Geometry check sheet. Reference: the model listing, model coordinates, mm. Face numbers are marked on the shaded views. A direction names the side the tool comes from. Round coordinates to 2 decimals unless told otherwise and drop trailing zeros. Order: outer loops, then holes, each group sorted by start corner. A loop starts at its lowest first (then second) coordinate and runs counter-clockwise, first axis right, second up. Notation, with made-up numbers: (41, 63.25) - (84, 63.25) arc R16 cw to (84, 77.25) - close; hole circle Ø1 at (62.5, 80). An arc over 180 degrees is marked (long way). Return JSON: item names as keys, results as strings. Group by question number.
Q1. Sectioned sample at C-C, the plane y = -12. Record the cut outline in (x, z).
Q2. Gauge pin test, flat ends, axial feed: pin 1 Ø10 at (y, z) = (-6.5, 1.5) entering from +X; pin 2 Ø12 at (y, z) = (-9.5, -4) entering from +X; pin 3 Ø6 at (x, z) = (0, 10.5) entering from -Y. Record the tip position at first contact, or that the pin passes through.
Q3. Material ranges on line 1 along X through (y, z) = (6, 0); line 2 along X through (y, z) = (8.5, -9); line 3 along Z through (x, y) = (7, 5.5), recorded low to high.
Q4. Draft check along X on the marked faces 3, 4 and 5. Enter one of: pulls with the +X half, pulls with the -X half, needs draft (parallel to the pull), parting line crosses it, or undercut.
Q5. Tool access check on the marked faces 1 and 2. Record the directions out of +Z, -Z, +X, -X, +Y, -Y that give a thin tool (end or side, any length) a straight path to the whole face; none if there is none.
Q6. Sectioned sample at B-B, the plane x = 0. Record the cut outline in (y, z), then the cut area to 3 significant figures.
Q7. Sectioned sample at A-A, the plane z = 0. Record the cut outline in (x, y), then the cut area to 3 significant figures.
```python
from build123d import *


with BuildPart() as part:
    # Esquisse1 → Révolution1 (revolve)
    with BuildSketch(Plane.XY, mode=Mode.PRIVATE) as r_volution1_sk:
        with BuildLine():
            Line((-10, 0), (-10, 12.083333333))
            Line((-10, 12.083333333), (-12, 12.083333333))
            Line((-12, 12.083333333), (-12, 1.880668734))
            Line((-12, 1.880668734), (-14, 1.880668734))
            Line((-14, 1.880668734), (-9.459459459, -11.362574509))
            ThreePointArc((-9.459459459, -11.362574509), (-5.812381937, -16.256665978), (0, -18.119331266))
            Line((0, -18.119331266), (0, 0))
            Line((0, 0), (-10, 0))
        make_face()
    revolve(r_volution1_sk.sketch.rotate(Axis((0, 0, 0), (0, 1, 0)), 270), axis=Axis((0, 0, 0), (0, 1, 0)))


solid = part.part
```
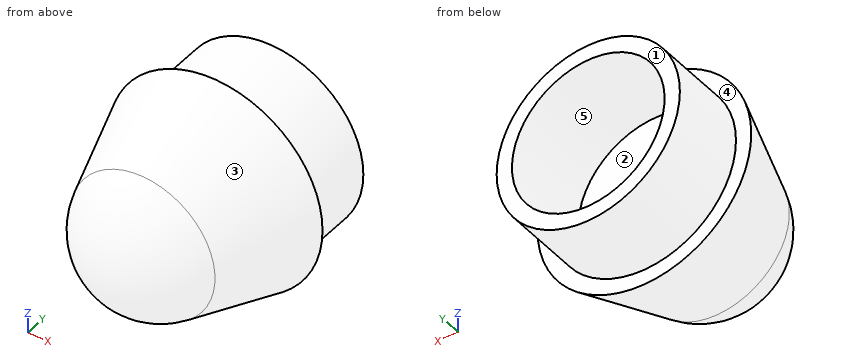
Reply:
{
 "1": {"outline": "circle Ø18.43 at (0, 0)"},
 "2": {"pin 1": "x = 12.8", "pin 2": "x = 11.88", "pin 3": "y = -14.73"},
 "3": {"line 1": "-12 to -10, 10 to 12", "line 2": "-7.94 to -4.36, 4.36 to 7.94", "line 3": "-9.75 to -7.14, 7.14 to 9.75"},
 "4": {"face 3": "parting line crosses it", "face 4": "needs draft", "face 5": "undercut"},
 "5": {"face 1": "+Z, -Z, +X, -X, +Y", "face 2": "+Y"},
 "6": {"outline": "(-11.36, -9.46) - (1.88, -14) - (1.88, -12) - (12.08, -12) - (12.08, -10) - (0, -10) - (0, 10) - (12.08, 10) - (12.08, 12) - (1.88, 12) - (1.88, 14) - (-11.36, 9.46) arc R10 ccw to start", "area": "407 mm^2"},
 "7": {"outline": "(-14, 1.88) - (-9.46, -11.36) arc R10 ccw to (9.46, -11.36) - (14, 1.88) - (12, 1.88) - (12, 12.08) - (10, 12.08) - (10, 0) - (-10, 0) - (-10, 12.08) - (-12, 12.08) - (-12, 1.88) - close", "area": "407 mm^2"}
}
